CAD build for the part. Positions are in the model's coordinates, mm. A direction names the side the tool comes from. Coordinates: 2 decimals unless noted, no trailing zeros. Write each loop counter-clockwise with the first axis right and the second up, starting at its lowest first coordinate (ties: lowest second). Pieces come first, ordered by that corner, then holes. Notation, with made-up numbers: (-12, 1.25) - (35, 1.25) arc R14 cw to (35, 25.25) - close; hole circle Ø5 at (81, 19). An arc over 180 degrees is marked (long way). Answer in a Markdown table with one row per item. Add a question column.
Q1. Drill centre lines: line 1 along Z through (x, y) = (0, 56.25); line 2 along Y through (x, z) = (9, 35). Where is each one in solid material? Low to high. Write a range as from..to.
Q2. Band-saw the part on D-D (z = 67.4). List the corners of the cut face in (x, y), and give its area (3 significant figures).
Q3. Band-saw the part on A-A (z = 52). List the corners of the cut face in (x, y), and give its area (3 significant figures).
Q4. Pin check, flat tip, straight feed: pin 1 (1.5 mm diameter, centred on x = 28.5, y = -22.5, fed in from +Z). Stop position of the tip, or through.
Q5. Two-plate mould, pull along Z, no slides. Class faces 3 (the cylindrical face through (-0.6, 57.46, 71.96)), 4 (the flat face through (60, 1, 37)), 5 (the flat face through (-5, -57, 80)), 6 (the cylindrical face through (57.54, 1.38, 63.01)): +Z half, -Z half, draft (parallel to the pull), parting line (faces both ways), or undercut.
Q6. 3-axis set-ups, long thin cutter, end or side, ignore diameter. For faces 1 (the cylindrical face through (-57.46, 1.38, 63.01)), 2 (the flat face through (55, 1, 39)): which of +Z, -Z, +X, -X, +Y, -Y reach the whole face in a straight line?
Q7. Band-saw the part on B-B (x = 0). List the corners of the cut face in (y, z).
Autodesk Inventor part; units mm, degrees
ref_plane "YZ Plane" through (0, 0, 0) normal (1, 0, 0) x (0, 1, 0)
ref_plane "XZ Plane" through (0, 0, 0) normal (0, 1, 0) x (-1, 0, 0)
ref_plane "XY Plane" through (0, 0, 0) normal (0, 0, 1) x (1, 0, 0)
sketch "Sketch1" plane through (0, 0, 0) normal (0, 0, 1) x (1, 0, 0)
  line L0 (-55, 55) -> (55, 55)
  line L1 (55, 55) -> (55, -55)
  line L2 (55, -55) -> (-55, -55)
  line L3 (-55, -55) -> (-55, 55)
  line L4 (-60, 60) -> (60, 60)
  line L5 (60, 60) -> (60, -60)
  line L6 (60, -60) -> (-60, -60)
  line L7 (-60, -60) -> (-60, 60)
  point P0 (0, 0)
  dimension "d0" = 110
  dimension "d1" = 110
  dimension "d2" = 55
  dimension "d3" = 55
  dimension "d4" = 5
  dimension "d5" = 5
  dimension "d6" = 5
  dimension "d7" = 5
extrude "Extrusion1" add sketch "Sketch1" along normal blind 80
sketch "Sketch2" plane through (0, 0, 0) normal (0, 0, -1) x (-1, 0, 0)
  line L0 (60, 60) -> (60, -60)
  line L1 (-60, 60) -> (60, 60)
  line L2 (60, 60) -> (60, -60)
  line L3 (60, -60) -> (-60, -60)
  line L4 (-60, -60) -> (-60, 60)
  point P0 (0, 0)
extrude "Extrusion2" add sketch "Sketch2" along normal blind 5
sketch "Sketch3" plane through (-60, -60, 80) normal (0, -1, 0) x (1, 0, 0)
  circle A0 centre (60, -12.6) radius 4.6
  line L0 (0, 0) -> (120, 0)
  line L1 (120, 0) -> (120, -85)
  point P0 (60, -80)
  dimension "d12" = 9.2
  dimension "d13" = 12.6
  dimension "d14" = 60
sketch "Sketch4" plane through (60, -60, 80) normal (1, 0, 0) x (0, 0, -1)
  circle A0 centre (12.6, 60) radius 4.6
  line L0 (0, 0) -> (0, 120)
  line L1 (0, 120) -> (85, 120)
  point P0 (60, -120)
  dimension "d15" = 9.2
  dimension "d18" = 12.6
  dimension "d19" = 60
extrude "Extrusion3" cut sketch "Sketch4" against normal blind 120
extrude "Extrusion4" cut sketch "Sketch3" against normal blind 120
equation "\"d1\" = d0"
equation "\"d5\" = d4"
equation "\"d6\" = d4"
equation "\"d7\" = d4"
properties part number "Box" material "ABS Plastic"
Checked values:
| question | item | result |
|---|---|---|
| 1 | line 1 | z = -5..62.8, 72..80 |
| 1 | line 2 | y = -60..-55, 55..60 |
| 2 | outline | (-60, -60) - (-4.6, -60) - (-4.6, -55) - (-55, -55) - (-55, -4.6) - (-60, -4.6) - close; (-60, 4.6) - (-55, 4.6) - (-55, 55) - (-4.6, 55) - (-4.6, 60) - (-60, 60) - close; (4.6, -60) - (60, -60) - (60, -4.6) - (55, -4.6) - (55, -55) - (4.6, -55) - close; (4.6, 55) - (55, 55) - (55, 4.6) - (60, 4.6) - (60, 60) - (4.6, 60) - close |
| 2 | area | 2,120 mm² |
| 3 | outline | (-60, -60) - (60, -60) - (60, 60) - (-60, 60) - close; hole (-55, -55) - (55, -55) - (55, 55) - (-55, 55) - close |
| 3 | area | 2,300 mm² |
| 4 | pin 1 | stops at z = 0 |
| 5 | face 3 | undercut |
| 5 | face 4 | draft |
| 5 | face 5 | +Z half |
| 5 | face 6 | undercut |
| 6 | face 1 | +X, -X |
| 6 | face 2 | +Z |
| 7 | outline | (-60, -5) - (60, -5) - (60, 62.8) - (55, 62.8) - (55, 0) - (-55, 0) - (-55, 62.8) - (-60, 62.8) - close; (-60, 72) - (-55, 72) - (-55, 80) - (-60, 80) - close; (55, 72) - (60, 72) - (60, 80) - (55, 80) - close |
